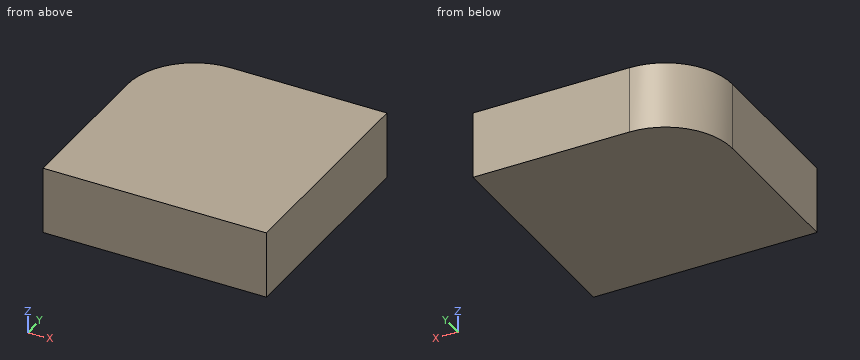
from build123d import *

# Parameters (mm, degrees)
BOSS_EXTRUDE1_DEPTH = 76.2


with BuildPart() as part:
    # Sketch1 → Boss-Extrude1 (new body)
    with BuildSketch(Plane.XY):
        with BuildLine():
            Line((0, 0), (0, 254))
            Line((0, 254), (-177.8, 254))
            ThreePointArc((-177.8, 254), (-231.681536726, 231.681536726), (-254, 177.8))
            Line((-254, 177.8), (-254, 0))
            Line((-254, 0), (0, 0))
        make_face()
    extrude(amount=-BOSS_EXTRUDE1_DEPTH)


solid = part.part
Input: part model. Units: mm. Frame: model coordinates. Give positions to 0.01 mm unless a question says otherwise; leave off trailing zeros. Loops run counter-clockwise (first coordinate to the right, second up) from the corner with the lowest first, then second, coordinate; pieces in that order, holes last. Notation, with made-up numbers: M -23,29 L 12,29 A15 ccw 12,53 Z; hole C 78.5,-28.5 d10. An arc over 180 degrees is marked long. Use one line per item in the form item = value.
1. Line query: L1, parallel to X at y = 201, z = -22.5; L2, parallel to Y at x = -188, z = -26; L3, parallel to Y at x = -208, z = -51.5. Output: solid intervals per line, ascending.
Numbers:
L1 = -250.38 to 0
L2 = 0 to 253.31
L3 = 0 to 247.76
2. Section query C-C, the plane x = -216. Return the cut outline in (y, z), and give its area (3 significant figures).
Numbers:
outline = M 0,-76.2 L 243.73,-76.2 L 243.73,0 L 0,0 Z
area = 18,600 mm²
3. Section query A-A, the plane z = -17. Return the cut outline in (x, y).
Numbers:
outline = M -254,0 L 0,0 L 0,254 L -177.8,254 A76.2 ccw -254,177.8 Z
4. Section query B-B, the plane y = 237.5. Return the cut outline in (x, z).
Numbers:
outline = M -225.15,-76.2 L 0,-76.2 L 0,0 L -225.15,0 Z
